from build123d import *

# Parameters (mm, degrees)
SKETCH_1_W          = 104
SKETCH_1_H          = 135
SKETCH_1_R          = 47
EXTRUDE_2_DEPTH     = 100
SKETCH_2_W          = 94
SKETCH_2_H          = 94
CUT_EXTRUDE_1_DEPTH = 95
SKETCH_3_W          = 30
SKETCH_3_H          = 5
SKETCH_3_W_2        = 94
SKETCH_3_H_2        = 20
CUT_EXTRUDE_3_DEPTH = 70
SKETCH_4_W          = 20
SKETCH_4_H          = 4
SKETCH_4_W_2        = 4
SKETCH_4_H_2        = 20
CUT_EXTRUDE_4_DEPTH = 10
CUT_EXTRUDE_6_REACH = 106
SKETCH_6_W          = 53.5
SKETCH_6_H          = 17
CUT_EXTRUDE_7_REACH = 137
SKETCH_7_W          = 12
SKETCH_7_H          = 12


with BuildPart() as part:
    # 草圖1 → 填料-伸長2 (new body)
    with BuildSketch(Plane.XY):
        with Locations((-20.894077044, -18.213740458)):
            Rectangle(SKETCH_1_W, SKETCH_1_H)
        with Locations((-20.894077044, -7.713740458)):
            Circle(SKETCH_1_R, mode=Mode.SUBTRACT)
    extrude(amount=EXTRUDE_2_DEPTH)

    # 草圖2 → 除料-伸長1 (cut)
    with BuildSketch(Plane.XY.offset(100)):
        with Locations((-20.894077044, -7.713740458)):
            Rectangle(SKETCH_2_W, SKETCH_2_H)
    extrude(amount=-CUT_EXTRUDE_1_DEPTH, mode=Mode.SUBTRACT)

    # 草圖3 → 除料-伸長3 (cut)
    with BuildSketch(Plane.XY.offset(100)):
        with Locations((11.105922956, -57.213740458)):
            Rectangle(SKETCH_3_W, SKETCH_3_H)
        with Locations((-20.894077044, -69.713740458)):
            Rectangle(SKETCH_3_W_2, SKETCH_3_H_2)
    extrude(amount=-CUT_EXTRUDE_3_DEPTH, mode=Mode.SUBTRACT)

    # 草圖4 → 除料-伸長4 (cut)
    with BuildSketch(Plane.XY.offset(100)):
        with Locations((-15.894077044, -81.713740458)):
            Rectangle(SKETCH_4_W, SKETCH_4_H)
        with Locations((28.105922956, -8.713740458)):
            Rectangle(SKETCH_4_W_2, SKETCH_4_H_2)
        with Locations((-15.894077044, 41.286259542)):
            Rectangle(SKETCH_4_W, SKETCH_4_H)
    extrude(amount=-CUT_EXTRUDE_4_DEPTH, mode=Mode.SUBTRACT)

    # 草圖6 → 除料-伸長6 (cut, up to next)
    with BuildSketch(Plane.ZY.offset(72.894077044), mode=Mode.PRIVATE) as cut_extrude_6_sk1:
        with Locations((63.25, 22.786259542)):
            Rectangle(SKETCH_6_W, SKETCH_6_H)
    cut_extrude_6_tool1 = extrude(cut_extrude_6_sk1.sketch, amount=-CUT_EXTRUDE_6_REACH, mode=Mode.PRIVATE) & part.part
    add(cut_extrude_6_tool1.solids().sort_by_distance((-72.894077, 22.78626, 63.25))[0], mode=Mode.SUBTRACT)
    # 草圖6 → 除料-伸長6 (cut, up to next)
    with BuildSketch(Plane.ZY.offset(72.894077044), mode=Mode.PRIVATE) as cut_extrude_6_sk2:
        with Locations((63.25, 1.786259542)):
            Rectangle(SKETCH_6_W, SKETCH_6_H)
    cut_extrude_6_tool2 = extrude(cut_extrude_6_sk2.sketch, amount=-CUT_EXTRUDE_6_REACH, mode=Mode.PRIVATE) & part.part
    add(cut_extrude_6_tool2.solids().sort_by_distance((-72.894077, 1.78626, 63.25))[0], mode=Mode.SUBTRACT)
    # 草圖6 → 除料-伸長6 (cut, up to next)
    with BuildSketch(Plane.ZY.offset(72.894077044), mode=Mode.PRIVATE) as cut_extrude_6_sk3:
        with Locations((63.25, -19.213740458)):
            Rectangle(SKETCH_6_W, SKETCH_6_H)
    cut_extrude_6_tool3 = extrude(cut_extrude_6_sk3.sketch, amount=-CUT_EXTRUDE_6_REACH, mode=Mode.PRIVATE) & part.part
    add(cut_extrude_6_tool3.solids().sort_by_distance((-72.894077, -19.21374, 63.25))[0], mode=Mode.SUBTRACT)
    # 草圖6 → 除料-伸長6 (cut, up to next)
    with BuildSketch(Plane.ZY.offset(72.894077044), mode=Mode.PRIVATE) as cut_extrude_6_sk4:
        with Locations((63.25, -40.213740458)):
            Rectangle(SKETCH_6_W, SKETCH_6_H)
    cut_extrude_6_tool4 = extrude(cut_extrude_6_sk4.sketch, amount=-CUT_EXTRUDE_6_REACH, mode=Mode.PRIVATE) & part.part
    add(cut_extrude_6_tool4.solids().sort_by_distance((-72.894077, -40.21374, 63.25))[0], mode=Mode.SUBTRACT)

    # 草圖7 → 除料-伸長7 (cut, up to next)
    with BuildSketch(Plane.XZ.offset(85.713740458), mode=Mode.PRIVATE) as cut_extrude_7_sk1:
        with Locations((5.105922956, 49)):
            Rectangle(SKETCH_7_W, SKETCH_7_H)
    cut_extrude_7_tool1 = extrude(cut_extrude_7_sk1.sketch, amount=-CUT_EXTRUDE_7_REACH, mode=Mode.PRIVATE) & part.part
    add(cut_extrude_7_tool1.solids().sort_by_distance((5.105923, -85.71374, 49))[0], mode=Mode.SUBTRACT)
    # 草圖7 → 除料-伸長7 (cut, up to next)
    with BuildSketch(Plane.XZ.offset(85.713740458), mode=Mode.PRIVATE) as cut_extrude_7_sk2:
        with Locations((-46.894077044, 49)):
            Rectangle(SKETCH_7_W, SKETCH_7_H)
    cut_extrude_7_tool2 = extrude(cut_extrude_7_sk2.sketch, amount=-CUT_EXTRUDE_7_REACH, mode=Mode.PRIVATE) & part.part
    add(cut_extrude_7_tool2.solids().sort_by_distance((-46.894077, -85.71374, 49))[0], mode=Mode.SUBTRACT)


solid = part.part
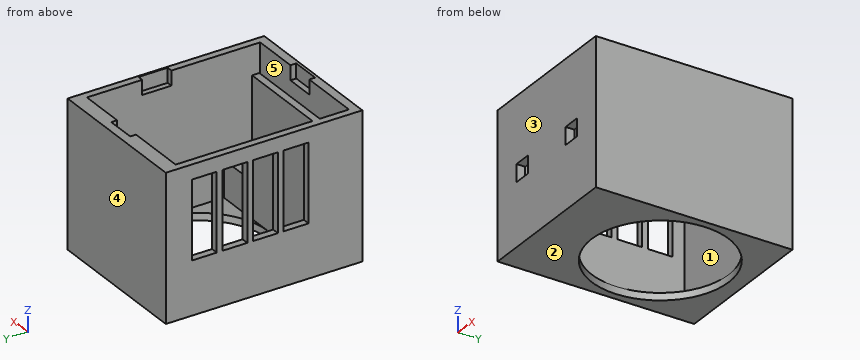
The model under review builds one solid part; all positions refer to its coordinate system, in mm. Face numbers are marked on the shaded views. A direction names the side the tool comes from. Coordinates: 2 decimals unless noted, no trailing zeros. Loops run counter-clockwise (first coordinate to the right, second up) from the corner with the lowest first, then second, coordinate; pieces in that order, holes last.
(1) Insertion check: P1, Ø3, axis at y = -37.5, z = 74, coming from the -X side; P2, Ø1.5, axis at x = -49.5, z = 51.5, coming from the -Y side; P3, Ø2, axis at x = 28, y = -4, coming from the +Z side. Each pin has a flat end and moves straight along its axis. Give the tip position at first contact, or say it passes through.
Determined:
P1: stops at x = 26.11
P2: stops at y = -59.71
P3: stops at z = 90
(2) Tool access review of the marked faces 4 and 5: name each direction out of +Z, -Z, +X, -X, +Y, -Y from which nothing blocks a thin tool from reaching the whole face with its end or side.
Determined:
face 4: +Z, -Z, +X, -X, +Y
face 5: +Z
(3) Consider section C-C, the plane x = 18. Give the boundary of the cut face in (y, z).
Determined:
outline: (-85.71, 0) - (-34.1, 0) - (-34.1, 5) - (-54.71, 5) - (-54.71, 30) - (-79.71, 30) - (-79.71, 100) - (-85.71, 100) - close; (18.67, 0) - (49.29, 0) - (49.29, 100) - (39.29, 100) - (39.29, 5) - (18.67, 5) - close
(4) Consider section D-D, the plane x = 5.5. Give the boundary of the cut face in (y, z).
Determined:
outline: (-85.71, 0) - (-46.6, 0) - (-46.6, 5) - (-54.71, 5) - (-54.71, 30) - (-79.71, 30) - (-79.71, 43) - (-85.71, 43) - close; (-85.71, 55) - (-79.71, 55) - (-79.71, 100) - (-85.71, 100) - close; (31.18, 0) - (49.29, 0) - (49.29, 100) - (39.29, 100) - (39.29, 5) - (31.18, 5) - close
(5) Consider section A-A, the plane z = 68. Give the boundary of the cut face in (x, y).
Determined:
outline: (-72.89, -85.71) - (31.11, -85.71) - (31.11, 49.29) - (-72.89, 49.29) - (-72.89, 31.29) - (-67.89, 31.29) - (-67.89, 39.29) - (26.11, 39.29) - (26.11, -79.71) - (-67.89, -79.71) - (-67.89, -59.71) - (-3.89, -59.71) - (-3.89, -54.71) - (-67.89, -54.71) - (-67.89, -48.71) - (-72.89, -48.71) - close; (-72.89, -31.71) - (-67.89, -31.71) - (-67.89, -27.71) - (-72.89, -27.71) - close; (-72.89, -10.71) - (-67.89, -10.71) - (-67.89, -6.71) - (-72.89, -6.71) - close; (-72.89, 10.29) - (-67.89, 10.29) - (-67.89, 14.29) - (-72.89, 14.29) - close
(6) Wall thickness on L1, parallel to Y at x = -59, z = 37; L2, parallel to Y at x = 22, z = 75.5; L3, parallel to Y at x = -22.5, z = 18.5: over which ranges is each line inside the solid? List them lowest first.
Determined:
L1: y = -85.71 to -79.71, -59.71 to -54.71, 39.29 to 49.29
L2: y = -85.71 to -79.71, 39.29 to 49.29
L3: y = -85.71 to -54.71, 39.29 to 49.29
(7) Draft analysis for pull direction Y (two halves, no side actions). For the marked faces 1, 2 and 3, state which applies: +Y half, -Y half, draft (parallel to the pull), parting line (faces both ways), or undercut.
Determined:
face 1: undercut
face 2: draft
face 3: -Y half
(8) Consider section B-B, the plane y = -66.5. Give the boundary of the cut face in (x, z).
Determined:
outline: (-72.89, 0) - (31.11, 0) - (31.11, 100) - (26.11, 100) - (26.11, 30) - (-67.89, 30) - (-67.89, 100) - (-72.89, 100) - close
